Here's how the part is built. I have some questions about the finished solid (model axes, mm). Coordinates: 2 decimals unless noted, no trailing zeros. Write each loop counter-clockwise with the first axis right and the second up, starting at its lowest first coordinate (ties: lowest second). Pieces come first, ordered by that corner, then holes. Notation, with made-up numbers: (59.5, 7) - (75.5, 7) arc R21 cw to (75.5, 38) - close; hole circle Ø7 at (35.25, 88.25). An arc over 180 degrees is marked (long way). Answer in a Markdown table with one row per item. Add a question column.
Item 1: Imagine slicing it at A-A (x = 0). Please give me the cut outline in (y, z), plus the area to 3 significant figures.
Item 2: If I drill on probe 1 along Z at (x, y) = (0, -0.6); probe 2 along X at (y, z) = (1.3, -1.5); probe 3 along Z at (x, y) = (-2.25, 1.05), over which ranges is the centre line in solid material (lowest first)? Write a range as from..to.
Item 3: Imagine slicing it at D-D (x = 4.25). Please give me the cut outline in (y, z).
Item 4: We'd pull the mould along Z, two halves only. Please class faces 1 (the face through (3.233, 0.021, -1.341)), 2 (the face through (0, 0, 5)), 3 (the face through (5, 0, -5)): +Z half, -Z half, draft (parallel to the pull), parting line (faces both ways), or undercut.
Item 5: Imagine slicing it at C-C (z = 2.5). Please give me the cut outline in (x, y).
Item 6: Imagine slicing it at B-B (y = 0.9). Please give me the cut outline in (x, z).
from build123d import *

# Parameters (mm, degrees)
F0_R     = 3.5
F1_DEPTH = 1.5


with BuildPart() as f1:
    # F0 (on Front) → F1 (new body, symmetric)
    with BuildSketch(Plane.XZ):
        with BuildLine():
            ThreePointArc((-5, 0), (0, -5), (5, 0))
            ThreePointArc((5, 0), (0, 5), (-5, 0))
        make_face()
        Circle(F0_R, mode=Mode.SUBTRACT)
        with BuildLine():
            Line((5, -10), (5, 0))
            ThreePointArc((5, 0), (0, -5), (-5, 0))
            Line((-5, 0), (-5, -10))
            Line((-5, -10), (5, -10))
        make_face()
    extrude(amount=F1_DEPTH, both=True)


solid = f1.part
Here are the results:
| question | item | result |
|---|---|---|
| 1 | outline | (-1.5, -10) - (1.5, -10) - (1.5, -3.5) - (-1.5, -3.5) - close; (-1.5, 3.5) - (1.5, 3.5) - (1.5, 5) - (-1.5, 5) - close |
| 1 | area | 24.0 mm2 |
| 2 | probe 1 | z = -10..-3.5, 3.5..5 |
| 2 | probe 2 | x = -5..-3.16, 3.16..5 |
| 2 | probe 3 | z = -10..-2.68, 2.68..4.47 |
| 3 | outline | (-1.5, -10) - (1.5, -10) - (1.5, 2.63) - (-1.5, 2.63) - close |
| 4 | face 1 | undercut |
| 4 | face 2 | +Z half |
| 4 | face 3 | draft |
| 5 | outline | (-4.33, -1.5) - (-2.45, -1.5) - (-2.45, 1.5) - (-4.33, 1.5) - close; (2.45, -1.5) - (4.33, -1.5) - (4.33, 1.5) - (2.45, 1.5) - close |
| 6 | outline | (-5, -10) - (5, -10) - (5, 0) arc R5 ccw to (-5, 0) - close; hole circle Ø7 at (0, 0) |
